from build123d import *

# Parameters (mm, degrees)
SKETCH1_R           = 19
SKETCH1_R_2         = 15
BOSS_EXTRUDE1_DEPTH = 3
BOSS_EXTRUDE2_DEPTH = 4
CUT_EXTRUDE1_DEPTH  = 4


with BuildPart() as part:
    # Sketch1 → Boss-Extrude1 (new body)
    with BuildSketch(Plane.XY):
        Polygon((5, -2.886751346), (5, 2.886751346), (0, 5.773502692), (-5, 2.886751346), (-5, -2.886751346), (0, -5.773502692), align=None)
        with BuildLine():
            Line((-4, 3.464101615), (0, 5.773502692))
            Line((0, 5.773502692), (4, 3.464101615))
            Line((4, 3.464101615), (4, 21.425824379))
            ThreePointArc((4, 21.425824379), (0, 21), (-4, 21.425824379))
            Line((-4, 21.425824379), (-4, 3.464101615))
        make_face()
        with Locations((0, 40)):
            Circle(SKETCH1_R)
        with Locations((0, 40)):
            Circle(SKETCH1_R_2, mode=Mode.SUBTRACT)
    extrude(amount=BOSS_EXTRUDE1_DEPTH)

    # Sketch2 → Boss-Extrude2 (add)
    with BuildSketch(Plane.XY.offset(3)):
        Polygon((0, -7.851963661), (6.8, -3.92598183), (6.8, 3.92598183), (0, 7.851963661), (-6.8, 3.92598183), (-6.8, -3.92598183), align=None)
        Polygon((0, -6.0044428), (5.2, -3.0022214), (5.2, 3.0022214), (0, 6.0044428), (-5.2, 3.0022214), (-5.2, -3.0022214), align=None, mode=Mode.SUBTRACT)
    extrude(amount=BOSS_EXTRUDE2_DEPTH)

    # Sketch3 → Cut-Extrude1 (cut, through all)
    with BuildSketch(Plane.XY.offset(3)):
        Polygon((4, 3.464101615), (4, 3.695041723), (0, 6.0044428), (-4, 3.695041723), (-4, 3.464101615), (-5, 2.886751346), (-5, -2.886751346), (0, -5.773502692), (5, -2.886751346), (5, 2.886751346), align=None)
    extrude(amount=-CUT_EXTRUDE1_DEPTH, mode=Mode.SUBTRACT)


solid = part.part
Part model, mm, in its own coordinate system. A direction names the side the tool comes from. Coordinates: 2 decimals unless noted, no trailing zeros. Loops run counter-clockwise (first coordinate to the right, second up) from the corner with the lowest first, then second, coordinate; pieces in that order, holes last. Notation, with made-up numbers: M 86,-30 L 98,-30 A31 cw 98,-4 Z; hole C 28,74 d9. An arc over 180 degrees is marked long. Use a Markdown table: item, result. Add a question column.
Q1. Which spindle directions (+Z, -Z, +X, -X, +Y, -Y) get a long thin tool onto all of the face, cutting with end or side? Do faces 4 (the flat face through (3.45, 5.86, 4.97)), 5 (the flat face through (-5.2, 0, 5)), 6 (the flat face through (-3.35, 5.92, 4.97)). Say none if no direction does.
Q2. Pin check, flat tips, straight feed: P1, Ø0.9, axis at y = 10.5, z = 2, coming from the +X side; P2, Ø19, axis at x = 4.5, y = 26.5, coming from the +Z side; P3, Ø2.5, axis at y = 15, z = 1.5, coming from the -X side; P4, Ø4, axis at x = 2, y = -2, coming from the -Z side. Stop position of each tip, or through.
Q3. Cut at B-B (x = -10). Write the cut outline in (y, z), and give its area (3 significant figures).
Q4. Cut at C-C (z = 4). Write the cut outline in (x, y), and give its area (3 significant figures).
Q5. Cut at A-A (y = 40). Write the cut outline in (x, z).
Q6. Probe L1, parallel to X at y = 2, z = 6.25; L2, parallel to Z at x = -6.5, y = 4; L3, parallel to Y at x = -1, z = 2.5. List the from-to ranges inside material, lowest first.
Q7. Mould opens along Y. For faces 1 (the cylindrical face through (0.779, 58.984, 1.479)), 2 (the flat face through (6.8, 0, 5)), 3 (the flat face through (5.2, 0, 5)) say: +Y half, -Y half, draft (parallel to the pull), parting line (faces both ways), or undercut.
Worked out:
| question | item | result |
|---|---|---|
| 1 | face 4 | +Z, +X, +Y |
| 1 | face 5 | +Z, -Z |
| 1 | face 6 | +Z, -X, +Y |
| 2 | P1 | stops at x = 4 |
| 2 | P2 | stops at z = 3 |
| 2 | P3 | stops at x = -4 |
| 2 | P4 | passes through |
| 3 | outline | M 23.84,0 L 28.82,0 L 28.82,3 L 23.84,3 Z; M 51.18,0 L 56.16,0 L 56.16,3 L 51.18,3 Z |
| 3 | area | 29.9 mm2 |
| 4 | outline | M -6.8,-3.93 L 0,-7.85 L 6.8,-3.93 L 6.8,3.93 L 0,7.85 L -6.8,3.93 Z; hole M -5.2,-3 L 0,-6 L 5.2,-3 L 5.2,3 L 0,6 L -5.2,3 Z |
| 4 | area | 66.5 mm2 |
| 5 | outline | M -19,0 L -15,0 L -15,3 L -19,3 Z; M 15,0 L 19,0 L 19,3 L 15,3 Z |
| 6 | L1 | x = -6.8 to -5.2, 5.2 to 6.8 |
| 6 | L2 | z = 3 to 7 |
| 6 | L3 | y = 5.43 to 25.03, 54.97 to 58.97 |
| 7 | face 1 | parting line |
| 7 | face 2 | draft |
| 7 | face 3 | undercut |
